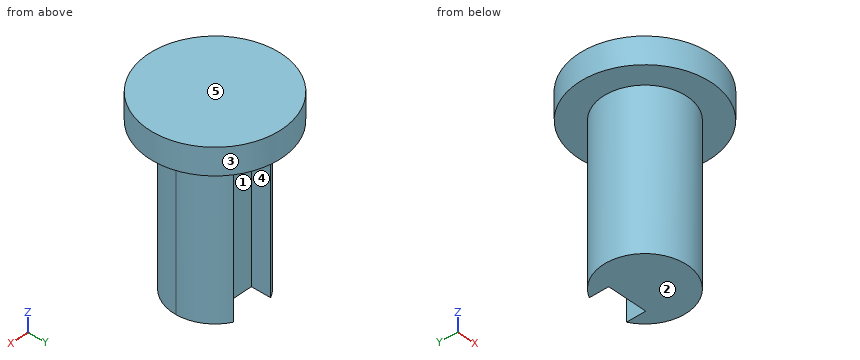
```python
from build123d import *

# Parameters (mm, degrees)
SKETCH1_R           = 15
BOSS_EXTRUDE1_DEPTH = 6
BOSS_EXTRUDE2_DEPTH = 35.2


with BuildPart() as part:
    # Sketch1 → Boss-Extrude1 (new body)
    with BuildSketch(Plane.XY):
        Circle(SKETCH1_R)
    extrude(amount=BOSS_EXTRUDE1_DEPTH)

    # Sketch1<3> → Boss-Extrude2 (add)
    with BuildSketch(Plane.XY):
        with BuildLine():
            Line((4.5, 8.366600265), (4.5, 4))
            Line((4.5, 4), (-4.5, 4))
            Line((-4.5, 4), (-4.5, 8.366600265))
            ThreePointArc((-4.5, 8.366600265), (-4.873397172, -8.154753215), (9.5, 0))
            ThreePointArc((9.5, 0), (8.154753215, 4.873397172), (4.5, 8.366600265))
        make_face()
    extrude(amount=-BOSS_EXTRUDE2_DEPTH)


solid = part.part
```
Source: CAD feature listing. Evaluate the final solid. Frame: model axes, mm. Face numbers are marked on the shaded views. A direction names the side the tool comes from. Give positions to 0.01 mm unless a question says otherwise; leave off trailing zeros. Loops run counter-clockwise (first coordinate to the right, second up) from the corner with the lowest first, then second, coordinate; pieces in that order, holes last. Notation, with made-up numbers: (6, 34) - (50, 34) arc R19 cw to (50, 57) - close; hole circle Ø4 at (22.5, 9.5). An arc over 180 degrees is marked (long way). Use CSV: the item, a comma, the result in double quotes. Start each with the question number.
1. Section B-B (y = 2.5). Output: boundary loops of the cut face in (x, z), then the cut area to 3 significant figures.
2. Section D-D (z = 1). Output: boundary loops of the cut face in (x, y), then the cut area to 3 significant figures.
3. Section C-C (z = -20.5). Output: boundary loops of the cut face in (x, y), then the cut area to 3 significant figures.
4. Pin query (flat end, axial travel): pin 1 (3.5 mm diameter, centred on y = 6.5, z = -24.5, fed in from -X); pin 2 (12 mm diameter, centred on x = 8, z = -0.5, fed in from +Y); pin 3 (8 mm diameter, centred on y = 8.5, z = -8, fed in from +X); pin 4 (12 mm diameter, centred on x = -6, y = 8.5, fed in from -Z). Return the tip coordinate at first contact, or that it passes through.
5. Reachability of the marked faces 1 and 2 from +Z, -Z, +X, -X, +Y, -Y: full face, straight path, thin tool, end or side. Return the list, or none.
6. Draft query along X for the marked faces 3, 4 and 5. Return one class per face: +X half, -X half, draft (parallel to the pull), parting line (faces both ways), or undercut.
7. Ray query, L1, parallel to Z at x = 9, y = -5.25; L2, parallel to X at y = 0.25, z = -20.5; L3, parallel to X at y = 6, z = -2.5. Return the intervals inside material, ascending.
8. Section A-A (x = 0). Output: boundary loops of the cut face in (y, z).
Response:
1,outline,"(-14.79, 0) - (-9.17, 0) - (-9.17, -35.2) - (9.17, -35.2) - (9.17, 0) - (14.79, 0) - (14.79, 6) - (-14.79, 6) - close"
1,area,"823 mm²"
2,outline,"circle Ø30 at (0, 0)"
2,area,"707 mm²"
3,outline,"(-4.5, 4) - (-4.5, 8.37) arc R9.5 ccw (long way) to (4.5, 8.37) - (4.5, 4) - close"
3,area,"237 mm²"
4,pin 1,"x = -8.23"
4,pin 2,"y = 14.86"
4,pin 3,"x = 8.37"
4,pin 4,"z = -35.2"
5,face 1,"-Z, +Y"
5,face 2,"-Z, +X, -X, +Y, -Y"
6,face 3,"parting line"
6,face 4,"undercut"
6,face 5,"draft"
7,L1,"0 to 6"
7,L2,"-9.5 to 9.5"
7,L3,"-7.37 to -4.5, 4.5 to 7.37"
8,outline,"(-15, 0) - (-9.5, 0) - (-9.5, -35.2) - (4, -35.2) - (4, 0) - (15, 0) - (15, 6) - (-15, 6) - close"
